from build123d import *

# Parameters (mm, degrees)
SALIENTE_EXTRUIR1_DEPTH = 100
CORTAR_EXTRUIR1_DEPTH   = 4
CROQUIS3_R              = 2.5
CORTAR_EXTRUIR2_DEPTH   = 14


with BuildPart() as part:
    # Croquis1 → Saliente-Extruir1 (new body)
    with BuildSketch(Plane.XY):
        with BuildLine():
            Line((-47.556708367, 5.923922341), (-25.353105055, 5.923922341))
            ThreePointArc((-25.353105055, 5.923922341), (-36.454906711, 14.423922341), (-47.556708367, 5.923922341))
        make_face()
    extrude(amount=SALIENTE_EXTRUIR1_DEPTH)

    # Croquis2 → Cortar-Extruir1 (cut)
    with BuildSketch(Plane.XZ.offset(-5.923922341)):
        Polygon((-36.454906711, 80.381197846), (-32.454906711, 82.690598923), (-32.454906711, 87.309401077), (-36.454906711, 89.618802154), (-40.454906711, 87.309401077), (-40.454906711, 82.690598923), align=None)
        Polygon((-36.454906711, 10.381197846), (-32.454906711, 12.690598923), (-32.454906711, 17.309401077), (-36.454906711, 19.618802154), (-40.454906711, 17.309401077), (-40.454906711, 12.690598923), align=None)
    extrude(amount=-CORTAR_EXTRUIR1_DEPTH, mode=Mode.SUBTRACT)

    # Croquis3 → Cortar-Extruir2 (cut)
    with BuildSketch(Plane.XZ.offset(-9.923922341)):
        with Locations((-36.454906711, 15)):
            Circle(CROQUIS3_R)
        with Locations((-36.454906711, 85)):
            Circle(CROQUIS3_R)
    extrude(amount=-CORTAR_EXTRUIR2_DEPTH, mode=Mode.SUBTRACT)


solid = part.part
Work out the finished part from the listing and answer in its coordinate system (mm). A direction names the side the tool comes from. Round coordinates to 2 decimals unless told otherwise and drop trailing zeros. Write each loop counter-clockwise with the first axis right and the second up, starting at its lowest first coordinate (ties: lowest second). Pieces come first, ordered by that corner, then holes.
1) Given pin 1 Ø4 at (x, z) = (-35, 85) entering from -Y; pin 2 Ø4.5 at (y, z) = (8.5, 14.5) entering from +X; pin 3 Ø12 at (x, z) = (-38.5, 60) entering from +Y; pin 4 Ø3 at (y, z) = (8.5, 15) entering from -X, each flat-ended and moving along its own axis, determine where each tip first touches the part or whether it passes through.
2) Straight lines are drawn through the part: line 1 (Z direction, x = -39.75, y = 8.5); line 2 (Z direction, x = -34.25, y = 11.25); line 3 (Y direction, x = -37, z = 40.5). For each, find the intervals that lie inside material, in ascending order.
3) A tool of negligible diameter and unlimited length cuts with its end or side. For faces 4 (the cylindrical face through (-34.07, 12.15, 85.75)), 5 (the flat face through (-38.48, 7.9, 11.55)), from which of +Z, -Z, +X, -X, +Y, -Y can it reach the whole face along a straight path? Write none if from no direction.
4) A cutting plane is placed at A-A (z = 15). Give the vertices of the cut face in (x, y), plus the area to 3 significant figures.
5) The mould has two halves that part along X. Classify faces 1 (the flat face through (-37, 5.924, 49)), 2 (the cylindrical face through (-36.24, 14.42, 49.3)), 3 (the flat face through (-38.43, 7.9, 18.48)): pulls with the +X half, pulls with the -X half, needs draft (parallel to the pull), parting line crosses it, or undercut.
6) A cutting plane is placed at D-D (x = -31). Give the vertices of the cut face in (y, z), plus the area to 3 significant figures.
7) A cutting plane is placed at C-C (z = 79). Give the vertices of the cut face in (x, y), plus the area to 3 significant figures.
8) A cutting plane is placed at B-B (y = 7.75). Give the vertices of the cut face in (x, z), plus the area to 3 significant figures.
Completed:
1. pin 1: stops at y = 9.92
1. pin 2: stops at x = -25.45
1. pin 3: stops at y = 14.42
1. pin 4: stops at x = -47.21
2. line 1: z = 0 to 12.28, 17.72 to 82.28, 87.72 to 100
2. line 2: z = 0 to 13.82, 16.18 to 83.82, 86.18 to 100
2. line 3: y = 5.92 to 14.41
3. face 4: +Y, -Y
3. face 5: -Y
4. outline: (-47.56, 5.92) - (-40.45, 5.92) - (-40.45, 9.92) - (-38.95, 9.92) - (-38.95, 14.15) arc R11.5 ccw to start; (-33.95, 9.92) - (-32.45, 9.92) - (-32.45, 5.92) - (-25.35, 5.92) arc R11.5 ccw to (-33.95, 14.15) - close
4. area: 85.5 mm2
5. face 1: needs draft
5. face 2: parting line crosses it
5. face 3: undercut
6. outline: (5.92, 0) - (13.05, 0) - (13.05, 100) - (5.92, 100) - close
6. area: 712 mm2
7. outline: (-47.56, 5.92) - (-25.35, 5.92) arc R11.5 ccw to start
7. area: 140 mm2
8. outline: (-46.89, 0) - (-26.02, 0) - (-26.02, 100) - (-46.89, 100) - close; hole (-40.45, 12.69) - (-36.45, 10.38) - (-32.45, 12.69) - (-32.45, 17.31) - (-36.45, 19.62) - (-40.45, 17.31) - close; hole (-40.45, 82.69) - (-36.45, 80.38) - (-32.45, 82.69) - (-32.45, 87.31) - (-36.45, 89.62) - (-40.45, 87.31) - close
8. area: 1,980 mm2
